```python
from build123d import *

# Parameters (mm, degrees)
BOSS_EXTRU_1_DEPTH      = 28
ESQUISSE2_R             = 7.5
BOSS_EXTRU_2_DEPTH      = 16
ESQUISSE3_R             = 16
BOSS_EXTRU_3_DEPTH      = 7.5
CHANFREIN2_SIZE2        = 5.251556537
CHANFREIN2_SIZE         = 7.5
ESQUISSE4_R             = 1.25
ENL_V_MAT_EXTRU_1_DEPTH = 7.5
ESQUISSE5_W             = 40
ESQUISSE5_H             = 40
ESQUISSE5_R             = 18.9
ESQUISSE5_R_2           = 10
BOSS_EXTRU_4_DEPTH      = 9
ESQUISSE7_W             = 14.5
ESQUISSE7_H             = 7
ENL_V_MAT_EXTRU_2_DEPTH = 9
ESQUISSE8_W             = 3
ESQUISSE8_H             = 10
ENL_V_MAT_EXTRU_3_DEPTH = 9
ESQUISSE9_R             = 3
ESQUISSE9_W             = 3
ESQUISSE9_H             = 6.5
ENL_V_MAT_EXTRU_4_DEPTH = 9
CONG_2_R                = 5


# Some blends are built 0.0001 mm under size
with BuildPart() as part:
    # Esquisse1 → Boss.-Extru.1 (new body)
    with BuildSketch(Plane.XY):
        with BuildLine():
            Line((-27, 0), (27, 0))
            Line((27, 0), (27, 49))
            ThreePointArc((27, 49), (0, 46), (-27, 49))
            Line((-27, 49), (-27, 0))
        make_face()
    extrude(amount=BOSS_EXTRU_1_DEPTH)

    # Esquisse2 → Boss.-Extru.2 (add)
    with BuildSketch(Plane.XY.offset(28)):
        with Locations((-11, 29)):
            Circle(ESQUISSE2_R)
    extrude(amount=BOSS_EXTRU_2_DEPTH)

    # Esquisse3 → Boss.-Extru.3 (add)
    with BuildSketch(Plane.XY.offset(28)):
        with Locations(Location((-11, 29, 0), (0, 0, 180))):
            Circle(ESQUISSE3_R)
    extrude(amount=BOSS_EXTRU_3_DEPTH)

    # Chanfrein2
    chanfrein2_edges = [part.edges().sort_by_distance(p)[0] for p in [
        (5, 29, 35.5),
    ]]
    chanfrein2_side = [part.faces().sort_by_distance(p)[0] for p in [
        (5, 29, 35.394968869),
    ]]
    chamfer(chanfrein2_edges, length=CHANFREIN2_SIZE - 0.0001, length2=CHANFREIN2_SIZE2 - 0.0001, reference=chanfrein2_side[0])  # a hair under: the kernel refuses the full size

    # Esquisse4 → Enlèv. mat.-Extru.1 (cut)
    with BuildSketch(Plane.XZ):
        with Locations(Location((-13, 5.5, 0), (0, 0, 270))):
            Circle(ESQUISSE4_R)
        with Locations(Location((13, 5.5, 0), (0, 0, 270))):
            Circle(ESQUISSE4_R)
    extrude(amount=-ENL_V_MAT_EXTRU_1_DEPTH, mode=Mode.SUBTRACT)

    # Esquisse5 → Boss.-Extru.4 (add)
    # profile 1 of 2: a face of its own
    with BuildSketch(Plane(origin=(0, 0, 0), x_dir=(-1, 0, 0), z_dir=(0, 0, -1))):
        with Locations((0, 23.4)):
            Rectangle(ESQUISSE5_W, ESQUISSE5_H)
        with Locations((0, 23.4)):
            Circle(ESQUISSE5_R, mode=Mode.SUBTRACT)
    # profile 2 of 2: a face of its own
    with BuildSketch(Plane(origin=(0, 0, 0), x_dir=(-1, 0, 0), z_dir=(0, 0, -1))):
        with Locations(Location((0, 23.4, 0), (0, 0, 180))):
            Circle(ESQUISSE5_R_2)
    extrude(amount=BOSS_EXTRU_4_DEPTH)

    # Esquisse7 → Enlèv. mat.-Extru.2 (cut)
    with BuildSketch(Plane(origin=(0, 49, 0), x_dir=(1, 0, 0), z_dir=(0, 1, 0))):
        with Locations((-14, -6.7)):
            Rectangle(ESQUISSE7_W, ESQUISSE7_H)
        with Locations((14, -6.7)):
            Rectangle(ESQUISSE7_W, ESQUISSE7_H)
    extrude(amount=-ENL_V_MAT_EXTRU_2_DEPTH, mode=Mode.SUBTRACT)

    # Esquisse8 → Enlèv. mat.-Extru.3 (cut)
    with BuildSketch(Plane.ZY.offset(27)):
        with BuildLine():
            Line((14.6, 27), (14.6, 20.5))
            Line((14.6, 20.5), (16.6, 20.5))
            ThreePointArc((16.6, 20.5), (17.307106781, 20.792893219), (17.6, 21.5))
            Line((17.6, 21.5), (17.6, 26))
            ThreePointArc((17.6, 26), (17.307106781, 26.707106781), (16.6, 27))
            Line((16.6, 27), (14.6, 27))
        make_face()
        with Locations((16.1, 34)):
            Rectangle(ESQUISSE8_W, ESQUISSE8_H)
    extrude(amount=-ENL_V_MAT_EXTRU_3_DEPTH, mode=Mode.SUBTRACT)

    # Esquisse9 → Enlèv. mat.-Extru.4 (cut)
    with BuildSketch(Plane(origin=(27, 0, 0), x_dir=(0, 0, -1), z_dir=(1, 0, 0))):
        with Locations(Location((-8, 11, 0), (0, 0, 90))):
            Circle(ESQUISSE9_R)
        with BuildLine():
            Line((-17.6, 39.1), (-17.6, 32.3))
            Line((-17.6, 32.3), (-16.047354824, 32.3))
            Line((-16.047354824, 32.3), (-14.673616115, 31.8))
            ThreePointArc((-14.673616115, 31.8), (-13.941138851, 31.896432461), (-13.6, 32.551754097))
            Line((-13.6, 32.551754097), (-13.6, 38.848245903))
            ThreePointArc((-13.6, 38.848245903), (-13.941138851, 39.503567539), (-14.673616115, 39.6))
            Line((-14.673616115, 39.6), (-16.047354824, 39.1))
            Line((-16.047354824, 39.1), (-17.6, 39.1))
        make_face()
        with Locations((-16.1, 23.95)):
            Rectangle(ESQUISSE9_W, ESQUISSE9_H)
    extrude(amount=-ENL_V_MAT_EXTRU_4_DEPTH, mode=Mode.SUBTRACT)

    # Congé2
    # the kernel refuses this fillet: 5 mm, written as the material it takes off along each edge
    with BuildSketch(Plane(origin=(20, 3.4, 0), x_dir=(-1, 0, 0), z_dir=(0, 0, -1)), Plane(origin=(-20, 3.4, 0), x_dir=(0, 1, 0), z_dir=(0, 0, -1)), Plane(origin=(20, 43.4, 0), x_dir=(0, -1, 0), z_dir=(0, 0, -1))) as cong_2_piece_1:
        with BuildLine():
            CenterArc((CONG_2_R, CONG_2_R), CONG_2_R, 180, 90)
            Line((0, CONG_2_R), (0, 0))
            Line((0, 0), (CONG_2_R, 0))
        make_face()
    extrude(amount=21.5, mode=Mode.SUBTRACT)
    with BuildSketch(Plane(origin=(-20, 43.4, 0), x_dir=(0, -1, 0), z_dir=(0, 0, -1))) as cong_2_piece_2:
        with BuildLine():
            CenterArc((CONG_2_R, -CONG_2_R), CONG_2_R, 90, 90)
            Line((0, -CONG_2_R), (0, 0))
            Line((0, 0), (CONG_2_R, 0))
        make_face()
    extrude(amount=21.5, mode=Mode.SUBTRACT)
    with BuildSketch(Plane(origin=(-27, 49, -15.238005323), x_dir=(0.9806535629636468, -0.19575134596396773, 0), z_dir=(0, 0, 1))) as cong_2_piece_3:
        with BuildLine():
            CenterArc((6.096411836, -4.998524955), CONG_2_R, 91.391765025, 99.896853443)
            Line((1.193144021, -5.977281685), (0, 0))
            ThreePointArc((0, 0), (2.987484684, -0.036286103), (5.974969369, 0))
        make_face()
    extrude(amount=58.476010646, mode=Mode.SUBTRACT)
    with BuildSketch(Plane(origin=(-27, 0, -12.5), x_dir=(1, 0, 0), z_dir=(0, 0, 1)), Plane(origin=(27, 0, -12.5), x_dir=(0, 1, 0), z_dir=(0, 0, 1))) as cong_2_piece_4:
        with BuildLine():
            CenterArc((CONG_2_R, CONG_2_R), CONG_2_R, 180, 90)
            Line((0, CONG_2_R), (0, 0))
            Line((0, 0), (CONG_2_R, 0))
        make_face()
    extrude(amount=53, mode=Mode.SUBTRACT)
    with BuildSketch(Plane(origin=(27, 49, -15.238005323), x_dir=(-0.9806535629636471, -0.19575134596396557, 0), z_dir=(0, 0, 1))) as cong_2_piece_5:
        with BuildLine():
            CenterArc((6.096411836, 4.998524955), CONG_2_R, 168.711381533, 99.896853443)
            Line((1.193144021, 5.977281685), (0, 0))
            ThreePointArc((0, 0), (2.987484684, 0.036286103), (5.974969369, 0))
        make_face()
    extrude(amount=58.476010646, mode=Mode.SUBTRACT)


solid = part.part
```
Geometry check sheet. Reference: the model listing, model coordinates, mm. A direction names the side the tool comes from. Give positions to 0.01 mm unless a question says otherwise; leave off trailing zeros. Loops run counter-clockwise (first coordinate to the right, second up) from the corner with the lowest first, then second, coordinate; pieces in that order, holes last. Notation, with made-up numbers: M -28,-37.75 L -4,-37.75 A28 cw -4,-9.75 Z; hole C -4.5,78.5 d5. An arc over 180 degrees is marked long. Write item = value, one per line.
(1) Release check for a two-part mould opening along Z. For faces 5 (the face through (25, 1, 14)), 6 (the face through (23, 27.2, 16)), 7 (the face through (-13.24, 21.68, 35.5)) record: released by +Z, released by -Z, zero draft, split by the parting line, or undercut.
Answer below:
face_5 = zero draft
face_6 = undercut
face_7 = released by +Z
(2) Tool access check on faces 1 (the face through (22.563, 39.354, 15.351)), 2 (the face through (0, 43.4, -4)), 3 (the face through (-18.5, 4.83, -4.44)), 4 (the face through (14.24, 3.7, 5.66)). Record the directions out of +Z, -Z, +X, -X, +Y, -Y that give a thin tool (end or side, any length) a straight path to the whole face; none if there is none.
Answer below:
face_1 = +X
face_2 = -Z, +X, -X, +Y
face_3 = -Z, -X, -Y
face_4 = -Y
(3) Material ranges on line 1 (Y direction, x = 23, z = 17); line 2 (Z direction, x = 22.25, y = 11); line 3 (X direction, y = 4.5, z = 5.5), recorded low to high. Write a range as [from, to].
Answer below:
line_1 = [0.1, 20.7], [27.2, 32.3], [39.1, 47.8]
line_2 = [0, 5], [11, 28]
line_3 = [-26.97, -14.25], [-11.75, 11.75], [14.25, 26.97]
(4) Sectioned sample at D-D, the plane x = 7.5. Record the cut outline in (y, z), plus the area to 3 significant figures.
Answer below:
outline = M 0,0 L 3.4,0 L 3.4,-9 L 6.05,-9 L 6.05,0 L 16.79,0 L 16.79,-9 L 30.01,-9 L 30.01,0 L 40.75,0 L 40.75,-9 L 43.4,-9 L 43.4,0 L 46.23,0 L 46.23,3.2 L 40,3.2 L 40,10.2 L 46.23,10.2 L 46.23,28 L 0,28 Z
area = 1,420 mm2
(5) Sectioned sample at B-B, the plane y = 11. Record the cut outline in (x, z).
Answer below:
outline = M -27,0 L -20,0 L -20,-9 L -14.26,-9 L -14.26,0 L 14.26,0 L 14.26,-9 L 20,-9 L 20,0 L 27,0 L 27,5 L 18,5 L 18,11 L 27,11 L 27,28 L -27,28 Z
(6) Sectioned sample at A-A, the plane z = 26. Record the cut outline in (x, y), plus the area to 3 significant figures.
Answer below:
outline = M -27,5 A5 ccw -22,0 L 22,0 A5 ccw 27,5 L 27,42.9 A5 ccw 21.14,47.83 A123 cw -21.14,47.83 A5 ccw -27,42.9 Z
area = 2,510 mm2
(7) Gauge pin test, flat ends, axial feed: pin 1 Ø8 at (y, z) = (30.5, 35) entering from -X; pin 2 Ø1 at (x, z) = (-15, 38) entering from +Y; pin 3 Ø3.5 at (x, y) = (22.5, 36.5) entering from -Z. Record the tip position at first contact, or that the pin passes through.
Answer below:
pin_1 = -24.84
pin_2 = 35.63
pin_3 = 0
